Verification items for the finished model (mm, model axes). A direction names the side the tool comes from. Round coordinates to 2 decimals unless told otherwise and drop trailing zeros. Write each loop counter-clockwise with the first axis right and the second up, starting at its lowest first coordinate (ties: lowest second). Pieces come first, ordered by that corner, then holes. Notation, with made-up numbers: (5, 63.25) - (16, 63.25) arc R26 cw to (16, 100.25) - close; hole circle Ø3 at (33, -33). An arc over 180 degrees is marked (long way). Write each question's results on one line, items separated by ' | '.
```python
from build123d import *

# Parameters (mm, degrees)
F0_W     = 53
F0_H     = 40
F1_DEPTH = 50
F2_W     = 37
F2_H     = 24
F3_DEPTH = 42
F4_W     = 8
F4_H     = 16
F5_DEPTH = 8


with BuildPart() as f1:
    # F0 (on Top) → F1 (new body)
    with BuildSketch(Plane.XY):
        with Locations((26.5, 20)):
            Rectangle(F0_W, F0_H)
    extrude(amount=F1_DEPTH)

    # F2 (on face) → F3 (cut)
    with BuildSketch(Plane.XY.offset(50)):
        with Locations((26.5, 20)):
            Rectangle(F2_W, F2_H)
    extrude(amount=-F3_DEPTH, mode=Mode.SUBTRACT)

    # F4 (on face) → F5 (cut, through all)
    with BuildSketch(Plane.YZ.offset(53)):
        with Locations((28, 16)):
            Rectangle(F4_W, F4_H)
    extrude(amount=-F5_DEPTH, mode=Mode.SUBTRACT)


solid = f1.part
```
(1) Section check A-A (z = 26). Record the cut outline in (x, y).
Answer:
outline: (0, 0) - (53, 0) - (53, 40) - (0, 40) - close; hole (8, 8) - (45, 8) - (45, 32) - (8, 32) - close
(2) Section check D-D (z = 15.5). Record the cut outline in (x, y), plus the area to 3 significant figures.
Answer:
outline: (0, 0) - (53, 0) - (53, 24) - (45, 24) - (45, 8) - (8, 8) - (8, 32) - (53, 32) - (53, 40) - (0, 40) - close | area: 1,170 mm2
(3) Mould release check, pull along Y, two halves, no side actions. Record for faces 4 (the flat face through (26, 0, 25)), 5 (the flat face through (26, 20, 0)), 6 (the flat face through (8, 20, 29)): released by +Y, released by -Y, zero draft, split by the parting line, or undercut.
Answer:
face 4: released by -Y | face 5: zero draft | face 6: undercut
(4) Section check C-C (y = 14). Record the cut outline in (x, z).
Answer:
outline: (0, 0) - (53, 0) - (53, 50) - (45, 50) - (45, 8) - (8, 8) - (8, 50) - (0, 50) - close
(5) Section check B-B (x = 48). Record the cut outline in (y, z), plus the area to 3 significant figures.
Answer:
outline: (0, 0) - (40, 0) - (40, 50) - (0, 50) - close; hole (24, 8) - (32, 8) - (32, 24) - (24, 24) - close | area: 1,870 mm2
(6) Set-up check for faces 1 (the flat face through (45, 20, 29)), 2 (the flat face through (53, 20, 25)), 3 (the flat face through (49, 24, 16)): record each of +Z, -Z, +X, -X, +Y, -Y from which the full face is reachable in a straight line by a thin tool's end or side.
Answer:
face 1: +Z | face 2: +Z, -Z, +X, +Y, -Y | face 3: +X
(7) Thickness scan on L1, parallel to X at y = 10.5, z = 24; L2, parallel to Y at x = 46.5, z = 9; L3, parallel to Y at x = 34.5, z = 34. Record the ranges inside material, lowest first.
Answer:
L1: 0 to 8, 45 to 53 | L2: 0 to 24, 32 to 40 | L3: 0 to 8, 32 to 40
